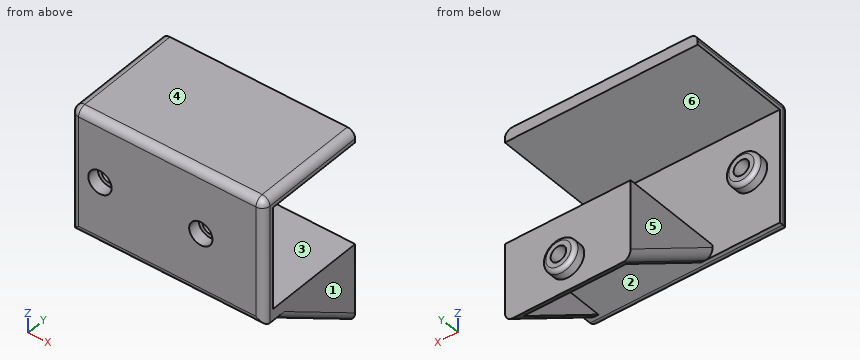
Autodesk Inventor part; units mm, degrees
ref_plane "YZ Plane" through (0, 0, 0) normal (1, 0, 0) x (0, 1, 0)
ref_plane "XZ Plane" through (0, 0, 0) normal (0, 1, 0) x (-1, 0, 0)
ref_plane "XY Plane" through (0, 0, 0) normal (0, 0, 1) x (1, 0, 0)
sketch "Sketch1" plane through (0, 0, 0) normal (0, 1, 0) x (-1, 0, 0)
  line L0 (20.5, 16.2) -> (-20.5, 16.2)
  line L1 (-20.5, 16.2) -> (-20.5, -16.2)
  line L2 (-20.5, -16.2) -> (20.5, -16.2)
  line L3 (20.5, -16.2) -> (20.5, 16.2)
  point P0 (0, 0)
  dimension "d0" = 41
  dimension "d1" = 32.4
extrude "Extrusion1" add sketch "Sketch1" along normal blind 3
sketch "Sketch4" plane through (20.5, 0, -16.2) normal (0, 0, -1) x (-1, 0, 0)
  line L0 (41, 3) -> (0, 3)
  line L1 (0, 28.4) -> (41, 28.4)
  line L2 (0, 3) -> (21.5, 3)
  line L3 (21.5, 3) -> (21.5, 28.4)
  line L4 (21.5, 28.4) -> (0, 28.4)
  line L5 (0, 28.4) -> (0, 3)
  point P0 (20.5, 0)
  dimension "d12" = 21.5
extrude "Extrusion4" cut sketch "Sketch4" against normal blind 3
sketch "Sketch5" plane through (-20.5, 0, 16.2) normal (0, 0, 1) x (1, 0, 0)
  line L0 (41, 28.4) -> (0, 28.4)
  line L1 (41, 3) -> (0, 3)
  line L2 (0, 28.4) -> (21.5, 28.4)
  line L3 (21.5, 28.4) -> (21.5, 3)
  line L4 (21.5, 3) -> (0, 3)
  line L5 (0, 3) -> (0, 28.4)
  point P0 (20.5, 0)
  point P1 (19.5, 3)
  point P2 (19.5, 3)
  dimension "d15" = 21.5
extrude "Extrusion5" cut sketch "Sketch5" against normal blind 3
sketch "Sketch6" plane through (0, 3, 0) normal (0, 1, 0) x (1, 0, 0)
  circle A0 centre (13, 0) radius 4.25
  circle A1 centre (-13, 0) radius 4.25
  point P0 (0, 0)
  dimension "d20" = 8.5
  dimension "d21" = 8.5
extrude "Extrusion6" add sketch "Sketch6" along normal blind 3
sketch "Sketch7" plane through (0, 0, 0) normal (0, -1, 0) x (1, 0, 0)
  circle A0 centre (-13, 0) radius 4.25
  circle A1 centre (-13, 0) radius 2
  circle A2 centre (13, 0) radius 4.25
  circle A3 centre (13, 0) radius 2
  point P0 (0, 0)
  dimension "d24" = 4
  dimension "d25" = 4
extrude "Extrusion7" cut sketch "Sketch7" against normal blind 6 contours A1 | A3
sketch "Sketch8" plane through (0, 0, 0) normal (0, -1, 0) x (1, 0, 0)
  circle A0 centre (-13, 0) radius 2
  circle A1 centre (-13, 0) radius 3
  circle A2 centre (13, 0) radius 2
  circle A3 centre (13, 0) radius 3
  point P0 (0, 0)
  dimension "d28" = 6
  dimension "d29" = 6
extrude "Extrusion8" cut sketch "Sketch8" against normal blind 3 contours A0 | A1 | A2 | A3
sketch "Sketch15" plane through (20.5, 0, 16.2) normal (1, 0, 0) x (0, 0, -1)
  line L0 (0, 3) -> (32.4, 3)
  line L1 (0, 0) -> (32.4, 0)
  line L2 (32.4, 0) -> (32.4, 3)
  line L3 (32.4, 3) -> (0, 3)
  line L4 (0, 3) -> (0, 0)
  point P0 (16.2, 0)
extrude "Extrusion15" add sketch "Sketch15" along normal blind 8.7
sketch "Sketch23" plane through (0, 3, 0) normal (0, 1, 0) x (1, 0, 0)
  line L0 (-20.5, 16.2) -> (29.2, 16.2)
  line L1 (29.2, 16.2) -> (-3.2, 16.2)
  line L2 (-3.2, 16.2) -> (-3.2, 13.2)
  line L3 (-3.2, 13.2) -> (29.2, 13.2)
  line L4 (29.2, 13.2) -> (29.2, 16.2)
  point P0 (0, 0)
  dimension "d81" = 32.4
  dimension "d82" = 3
extrude "Extrusion23" add sketch "Sketch23" along normal blind 26.4
sketch "Sketch24" plane through (-20.5, 0, -16.2) normal (0, 0, -1) x (-1, 0, 0)
  line L0 (-17.3, 3) -> (-17.3, 29.4)
  line L1 (-49.7, 3) -> (-17.3, 3)
  line L2 (-17.3, 29.4) -> (-20.3, 29.4)
  line L3 (-20.3, 29.4) -> (-20.3, 3)
  line L4 (-20.3, 3) -> (-17.3, 3)
  line L5 (-17.3, 3) -> (-17.3, 29.4)
  line L6 (-49.7, 0) -> (-49.7, 29.4)
  line L7 (-49.7, 29.4) -> (-46.7, 29.4)
  line L8 (-46.7, 29.4) -> (-46.7, 3)
  line L9 (-46.7, 3) -> (-49.7, 3)
  line L10 (-49.7, 3) -> (-49.7, 29.4)
  line L11 (-20.3, 29.4) -> (-46.7, 29.4)
  line L12 (-46.7, 29.4) -> (-46.7, 26.4)
  line L13 (-46.7, 26.4) -> (-20.3, 26.4)
  line L14 (-20.3, 26.4) -> (-20.3, 29.4)
  point P0 (-20.5, 0)
  dimension "d85" = 3
  dimension "d86" = 3
  dimension "d87" = 3
extrude "Extrusion24" add sketch "Sketch24" along normal blind 17.3 contours L1 L3 L2 L0 | L3 L13 L8 L11 | L1 L6 L7 L8
sketch "Sketch25" plane through (-3.2, 3, -13.2) normal (-1, 0, 0) x (0, 0, 1)
  line L0 (0, 26.4) -> (-20.3, 26.4)
  line L1 (0, 0) -> (-3, 0)
  line L2 (-20.3, 26.4) -> (-3, 0)
  line L3 (-20.3, 26.4) -> (-20.3, 0)
  line L4 (-3, 0) -> (-20.3, 0)
  line L5 (-20.3, 0) -> (-20.3, 26.4)
  point P0 (13.2, -3)
extrude "Extrusion25" cut sketch "Sketch25" against normal blind 32.4
sketch "Sketch26" plane through (0, 29.4, 0) normal (0, 1, 0) x (1, 0, 0)
  circle A0 centre (13, 26) radius 2
  point P0 (0, 0)
  dimension "d92" = 4
extrude "Extrusion26" cut sketch "Sketch26" against normal blind 32.4
sketch "Sketch27" plane through (0, 29.4, 0) normal (0, 1, 0) x (1, 0, 0)
  circle A0 centre (13, 26) radius 2
  circle A1 centre (13, 26) radius 4.25
  point P0 (0, 0)
  dimension "d95" = 8.5
extrude "Extrusion27" add sketch "Sketch27" along normal blind 3
sketch "Sketch28" plane through (0, 3, 0) normal (0, 1, 0) x (1, 0, 0)
  line L0 (-20.5, -16.2) -> (29.2, -16.2)
  line L1 (-20.5, 16.2) -> (-20.5, -16.2)
  line L2 (29.2, -16.2) -> (-20.5, -16.2)
  line L3 (-20.5, -16.2) -> (-20.5, -13.2)
  line L4 (-20.5, -13.2) -> (29.2, -13.2)
  line L5 (29.2, -13.2) -> (29.2, -16.2)
  point P0 (0, 0)
  dimension "d98" = 3
extrude "Extrusion28" add sketch "Sketch28" along normal blind 26.4
fillet "Fillet3" radius 1 3 edges at (8.75, 32.4, -26) (-17.25, 6, 0) (8.75, 6, 0)
fillet "Fillet4" radius 2 9 edges at (4.35, 0, 16.2) (-20.5, 0, 0) (29.2, 14.7, 16.2) (29.2, 0, 0) (29.2, 16.2, -24.85) (-3.2, 16.2, -24.85) (4.35, 0, -16.2) (13, 26.4, -31.5341) (-20.5, 14.7, 16.2)
sketch "Sketch29" plane through (-0.2, 26.4, -16.2) normal (0, -1, 0) x (1, 0, 0)
  circle A0 centre (13.2, -9.8) radius 2
  circle A1 centre (13.2, -9.8) radius 3
  point P0 (0.2, 16.2)
  dimension "d103" = 6
extrude "Extrusion29" cut sketch "Sketch29" against normal blind 3
properties part number "cornerMount_PBF"
Can you work these out from the model? Positions are in its coordinate system, mm. Face numbers are marked on the shaded views. A direction names the side the tool comes from. Coordinates: 2 decimals unless noted, no trailing zeros. Loops run counter-clockwise (first coordinate to the right, second up) from the corner with the lowest first, then second, coordinate; pieces in that order, holes last. Notation, with made-up numbers: (-33.75, 53) - (-28.75, 53) arc R10 cw to (-28.75, 67) - close; hole circle Ø5 at (56, 69). An arc over 180 degrees is marked (long way). Use a Markdown table: item, result.
Item 1: If I drill on probe 1 along Z at (x, y) = (13, 4); probe 2 along Z at (x, y) = (17.5, 26); probe 3 along X at (y, z) = (31, -26), over which ranges is the centre line in solid material (lowest first)? Write a range as from..to.
Numbers:
| item | result |
|---|---|
| probe 1 | z = -16.2..-13.2, -4.25..-2, 2..4.25, 13.2..16.2 |
| probe 2 | z = -16.2..-13.2, 13.2..16.2 |
| probe 3 | x = 8.75..11, 15..17.25 |
Item 2: I want a section at A-A on x = -13. Please give me the cut outline in (y, z), and give its area (3 significant figures).
Numbers:
| item | result |
|---|---|
| outline | (0, -14.2) arc R2 ccw to (2, -16.2) - (3, -16.2) - (3, -4.25) - (5, -4.25) arc R1 ccw to (6, -3.25) - (6, -2) - (3, -2) - (3, -3) - (0, -3) - close; (0, 3) - (3, 3) - (3, 2) - (6, 2) - (6, 3.25) arc R1 ccw to (5, 4.25) - (3, 4.25) - (3, 13.2) - (29.4, 13.2) - (29.4, 16.2) - (2, 16.2) arc R2 ccw to (0, 14.2) - close |
| area | 170 mm2 |
Item 3: Will these pins go through, and if not, where does the flat tip stop? pin 1 (3.5 mm diameter, centred on x = 13, z = 0, fed in from -Y); pin 2 (5 mm diameter, centred on x = -11.5, z = 0.5, fed in from +Y); pin 3 (5 mm diameter, centred on y = 11.5, z = -21, fed in from -X); pin 4 (8 mm diameter, centred on y = 12.5, z = -26, fed in from +X).
Numbers:
| item | result |
|---|---|
| pin 1 | passes through |
| pin 2 | stops at y = 6 |
| pin 3 | stops at x = -3.2 |
| pin 4 | stops at x = 28.94 |
Item 4: I want a section at B-B on z = 0. Give the number of separate pieces and of enclosed holes in the cut face, and give its area (3 significant figures).
Numbers:
| item | result |
|---|---|
| separate pieces | 3 |
| enclosed holes | 0 |
| area | 138 mm2 |
Item 5: I want a section at C-C on z = -12. Please give me the cut outline in (x, y), and give its area (3 significant figures).
Numbers:
| item | result |
|---|---|
| outline | (-20.5, 2) arc R2 ccw to (-18.5, 0) - (27.2, 0) arc R2 ccw to (29.2, 2) - (29.2, 3) - (-20.5, 3) - close |
| area | 147 mm2 |
Item 6: For the marked faces 1, 2 and 3, which set-ups out of +Z, -Z, +X, -X, +Y, -Y let a thin tool reach every point of the face, with its end or its side?
Numbers:
| item | result |
|---|---|
| face 1 | +Z, -Z, +X, +Y, -Y |
| face 2 | -Z, -Y |
| face 3 | +X, -X, +Y |
Item 7: We'd pull the mould along Z, two halves only. Please class the marked faces 4, 5 and 6: released by +Z, released by -Z, zero draft, split by the parting line, or undercut.
Numbers:
| item | result |
|---|---|
| face 4 | released by +Z |
| face 5 | zero draft |
| face 6 | undercut |
Item 8: I want a section at D-D on x = 22. Please give me the cut outline in (y, z), and give its area (3 significant figures).
Numbers:
| item | result |
|---|---|
| outline | (0, -14.2) arc R2 ccw to (2, -16.2) - (26.4, -16.2) - (26.4, -30.45) arc R2 ccw to (27.3, -32.13) - (29.4, -33.5) - (29.4, -13.2) - (3, -13.2) - (3, 13.2) - (29.4, 13.2) - (29.4, 16.2) - (2, 16.2) arc R2 ccw to (0, 14.2) - close |
| area | 303 mm2 |
